Part model, mm, in its own coordinate system. Give positions to 0.01 mm unless a question says otherwise; leave off trailing zeros. Order: outer loops, then holes, each group sorted by start corner. A loop starts at its lowest first (then second) coordinate and runs counter-clockwise, first axis right, second up. Notation, with made-up numbers: M 77.25,-37.75 L 100.25,-37.75 A10 ccw 100.25,-27.75 Z; hole C 88,36 d8. An arc over 180 degrees is marked long. Return JSON: item names as keys, results as strings.
from build123d import *

# Parameters (mm, degrees)
SKETCH1_R           = 8
BOSS_EXTRUDE1_DEPTH = 14
SKETCH2_W           = 16
SKETCH2_H           = 17.069791858
BOSS_EXTRUDE2_DEPTH = 7
SKETCH3_R           = 4
CUT_EXTRUDE1_DEPTH  = 29
SKETCH4_W           = 17.069791858
SKETCH4_H           = 7
CUT_EXTRUDE2_DEPTH  = 29


with BuildPart() as part:
    # Sketch1 → Boss-Extrude1 (new body)
    with BuildSketch(Plane(origin=(0, 0, 0), x_dir=(1, 0, 0), z_dir=(0, 1, 0))):
        Circle(SKETCH1_R)
    extrude(amount=BOSS_EXTRUDE1_DEPTH)

    # Sketch2 → Boss-Extrude2 (add)
    with BuildSketch(Plane(origin=(0, 14, 0), x_dir=(1, 0, 0), z_dir=(0, 1, 0))):
        Rectangle(SKETCH2_W, SKETCH2_H)
    extrude(amount=BOSS_EXTRUDE2_DEPTH)

    # Sketch3 → Cut-Extrude1 (cut)
    with BuildSketch(Plane.ZY.offset(8)):
        with Locations((0, 7)):
            Circle(SKETCH3_R)
    extrude(amount=-CUT_EXTRUDE1_DEPTH, mode=Mode.SUBTRACT)

    # Sketch4 → Cut-Extrude2 (cut)
    with BuildSketch(Plane.ZY.offset(8)):
        with Locations((0, 17.5)):
            Rectangle(SKETCH4_W, SKETCH4_H)
    extrude(amount=-CUT_EXTRUDE2_DEPTH, mode=Mode.SUBTRACT)


solid = part.part
Q1. Band-saw the part on D-D (x = 5.25). Give the cut face in (y, z).
Established:
{"outline": "M 0,-6.04 L 14,-6.04 L 14,6.04 L 0,6.04 Z; hole C 7,0 d8"}
Q2. Band-saw the part on B-B (x = 0). Give the cut face in (y, z), then the cut area to 3 significant figures.
Established:
{"outline": "M 0,-8 L 14,-8 L 14,8 L 0,8 Z; hole C 7,0 d8", "area": "174 mm²"}
Q3. Band-saw the part on C-C (y = 5.25). Give the cut face in (x, z), then the cut area to 3 significant figures.
Established:
{"outline": "M -7.15,-3.6 A8 ccw 7.15,-3.6 Z; M -7.15,3.6 L 7.15,3.6 A8 ccw Z", "area": "90.0 mm²"}
Q4. Probe line 1 along Y through (x, z) = (-2.25, 0); line 2 along Z through (x, y) = (1, 7); line 3 along Y through (x, z) = (-6.75, -3). List the from-to ranges inside material, lowest first.
Established:
{"line 1": "y = 0 to 3, 11 to 14", "line 2": "z = -7.94 to -4, 4 to 7.94", "line 3": "y = 0 to 4.35, 9.65 to 14"}
Q5. Band-saw the part on A-A (z = 0). Give the cut face in (x, y).
Established:
{"outline": "M -8,0 L 8,0 L 8,3 L -8,3 Z; M -8,11 L 8,11 L 8,14 L -8,14 Z"}
Q6. Pin check, flat tips, straight feed: pin 1 (4 mm diameter, centred on x = -2, y = 12.5, fed in from +Z); pin 2 (1.5 mm diameter, centred on y = 9.5, z = 3, fed in from -X); pin 3 (1.5 mm diameter, centred on y = 3, z = -5, fed in from +X); pin 4 (5 mm diameter, centred on x = 4, y = 8.5, fed in from -Z). Stop position of each tip, or through.
Established:
{"pin 1": "stops at z = 8", "pin 2": "stops at x = -7.59", "pin 3": "stops at x = 6.78", "pin 4": "stops at z = -7.86"}
Q7. Two-plate mould, pull along Z, no slides. Class faces 1 (the cylindrical face through (-6.349, 6.902, 4.868)), 2 (the cylindrical face through (-0.112, 5.468, 3.695)), 3 (the flat face through (0, 14, 0)): +Z half, -Z half, draft (parallel to the pull), parting line (faces both ways), or undercut.
Established:
{"face 1": "parting line", "face 2": "undercut", "face 3": "draft"}
